Geometry check sheet. Reference: the model listing, model coordinates, mm. Face numbers are marked on the shaded views. Round coordinates to 2 decimals unless told otherwise and drop trailing zeros. Order: outer loops, then holes, each group sorted by start corner. A loop starts at its lowest first (then second) coordinate and runs counter-clockwise, first axis right, second up.
(1) Sectioned sample at C-C (y = 6). Record the boundary of the cut face in (x, z), plus the area to 3 significant figures.
(2) Sectioned sample at A-A (x = 25). Record the boundary of the cut face in (y, z), plus the area to 3 significant figures.
(3) Material ranges on line 1 along Y through (x, z) = (25, 6.25); line 2 along Z through (x, y) = (5, 1.5); line 3 along X through (y, z) = (17.5, 1.75), recorded low to high.
(4) Sectioned sample at D-D (z = 4.5). Record the boundary of the cut face in (x, y).
(5) Sectioned sample at B-B (y = 2.5). Record the boundary of the cut face in (x, z), plus the area to 3 significant figures.
(6) Release check for a two-part mould opening along X. For the marked faces 1, 2 and 3 record: +X half, -X half, draft (parallel to the pull), parting line (faces both ways), or undercut.
(7) Go/stop test with flat-tipped pins: pin 1 (10 mm diameter, centred on x = 40.5, y = 11, fed in from +Z); pin 2 (8.5 mm diameter, centred on x = 41, y = 16, fed in from +Z); pin 3 (1.5 mm diameter, centred on x = 4.5, z = 4.5, fed in from -Y). Record where each tip stops, or that it passes through.
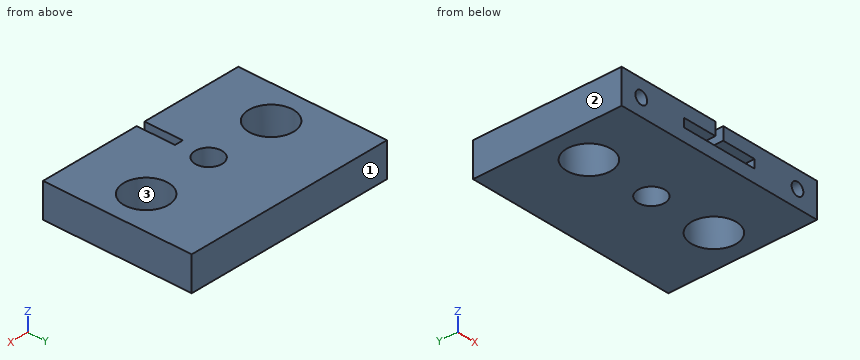
from build123d import *

# Parameters (mm, degrees)
F0_W     = 50
F0_H     = 35
F1_DEPTH = 8
F2_R     = 5.25
F2_R_2   = 3.15
F3_DEPTH = 8
F4_R     = 1.5
F5_DEPTH = 3
F6_DEPTH = 9


with BuildPart() as f1:
    # F0 (on Top) → F1 (new body)
    with BuildSketch(Plane.XY):
        with Locations((25, 17.5)):
            Rectangle(F0_W, F0_H)
    extrude(amount=F1_DEPTH)

    # F2 (on face) → F3 (cut)
    with BuildSketch(Plane.XY.offset(8)):
        with Locations((9, 16)):
            Circle(F2_R)
        with Locations((41, 16)):
            Circle(F2_R)
        with Locations((25, 16)):
            Circle(F2_R_2)
    extrude(amount=-F3_DEPTH, mode=Mode.SUBTRACT)

    # F4 (on face) → F5 (cut)
    with BuildSketch(Plane.XZ):
        with Locations((5, 4)):
            Circle(F4_R)
        with Locations((45, 4)):
            Circle(F4_R)
    extrude(amount=-F5_DEPTH, mode=Mode.SUBTRACT)

    # F4 (on face) → F6 (cut)
    with BuildSketch(Plane.XZ):
        Polygon((26, 8), (24, 8), (24, 5), (16, 5), (16, 3), (34, 3), (34, 5), (26, 5), align=None)
    extrude(amount=-F6_DEPTH, mode=Mode.SUBTRACT)


solid = f1.part
Answer below:
1. outline: (0, 0) - (50, 0) - (50, 8) - (26, 8) - (26, 5) - (34, 5) - (34, 3) - (16, 3) - (16, 5) - (24, 5) - (24, 8) - (0, 8) - close
1. area: 358 mm2
2. outline: (0, 0) - (12.85, 0) - (12.85, 8) - (9, 8) - (9, 3) - (0, 3) - close; (19.15, 0) - (35, 0) - (35, 8) - (19.15, 8) - close
2. area: 185 mm2
3. line 1: y = 9 to 12.85, 19.15 to 35
3. line 2: z = 0 to 2.5, 5.5 to 8
3. line 3: x = 0 to 3.97, 14.03 to 22.23, 27.77 to 35.97, 46.03 to 50
4. outline: (0, 0) - (3.59, 0) - (3.59, 3) - (6.41, 3) - (6.41, 0) - (16, 0) - (16, 9) - (34, 9) - (34, 0) - (43.59, 0) - (43.59, 3) - (46.41, 3) - (46.41, 0) - (50, 0) - (50, 35) - (0, 35) - close; hole circle Ø10.5 at (9, 16); hole circle Ø6.3 at (25, 16); hole circle Ø10.5 at (41, 16)
5. outline: (0, 0) - (50, 0) - (50, 8) - (26, 8) - (26, 5) - (34, 5) - (34, 3) - (16, 3) - (16, 5) - (24, 5) - (24, 8) - (0, 8) - close; hole circle Ø3 at (5, 4); hole circle Ø3 at (45, 4)
5. area: 344 mm2
6. face 1: draft
6. face 2: -X half
6. face 3: undercut
7. pin 1: stops at z = 8
7. pin 2: passes through
7. pin 3: stops at y = 3
